```python
from build123d import *


with BuildPart() as part:
    # Sketch → Revolution (revolve)
    with BuildSketch(Plane.XY):
        Polygon((-28.515713, 196), (28.515713, 196), (65.398537, 196), (73.283608, 201), (108, 201), (108, 216), (100, 216), (100, 207), (72.030521, 207), (63.161045, 201.026306), (-29.824583, 201.026306), (-78.099873, 201.026306), (-86.908587, 207), (-100, 207), (-100, 216), (-108, 216), (-108, 201), (-99.298126, 201), (-89.018097, 201), (-80.451416, 196), align=None)
    revolve(axis=Axis((0, 0, 0), (1, 0, 0)))

    # Sketch001 → Revolution001 (revolve)
    with BuildSketch(Plane.XZ):
        with BuildLine():
            Line((0, 0), (100.38707, 0))
            Line((100.38707, 0), (100.38707, 50.972863))
            ThreePointArc((100.38707, 50.972863), (98.816025, 73.680404), (89.94216, 94.641203))
            ThreePointArc((108.836403, 213.905151), (73.659034, 158.34946), (89.94216, 94.641203))
            Line((108.836403, 213.905151), (62.693928, 197.37645))
            Line((62.693928, 197.37645), (29.636631, 197.37645))
            ThreePointArc((29.636631, 197.37645), (34.494433, 122.49617), (51.28, 49.36))
            Line((51.28, 49.36), (0, 49.36))
            Line((0, 49.36), (0, 0))
        make_face()
    revolve(axis=Axis((0, 0, 0), (1, 0, 0)))


solid = part.part
```
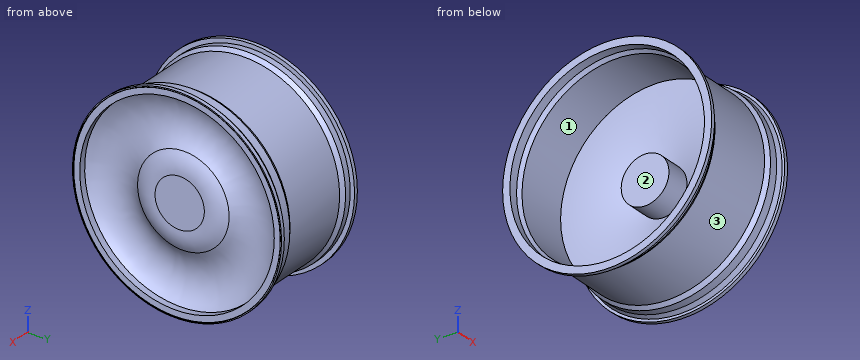
Model file for the job. Use its own axes, mm. Face numbers are marked on the shaded views. Round coordinates to 2 decimals unless told otherwise and drop trailing zeros. Loops run counter-clockwise (first coordinate to the right, second up) from the corner with the lowest first, then second, coordinate; pieces in that order, holes last. Notation, with made-up numbers: M 7.25,24.25 L 56.25,24.25 A22 ccw 56.25,58.25 Z; hole C 15,29 d2. An arc over 180 degrees is marked long. Put each result on its own line as item: value. Start each with the question number.
Item 1: Cut at A-A (x = -8.5). List the corners of the cut face in (y, z), then the cut area to 3 significant figures.
Item 2: Drill centre lines: line 1 along Z through (x, y) = (-95, 0); line 2 along Z through (x, y) = (103.75, 0); line 3 along Y through (x, z) = (-18.5, -141). Where is each one in solid material? Low to high.
Item 3: Drop flat-ended pins along their axis: P1, Ø3, axis at x = 4, z = -41, coming from the +Y side; P2, Ø3, axis at x = -9.5, y = 114.5, coming from the +Z side; P3, Ø2, axis at x = -71, y = -159.5, coming from the -Z side. Give the stop position or say it passes through.
Item 4: Mould opens along Z. For the marked faces 1, 2 and 3 say: released by +Z, released by -Z, zero draft, split by the parting line, or undercut.
Answer block:
1. outline: C 0,0 d402.05; hole C 0,0 d392
1. area: 6,270 mm2
2. line 1: -207 to -201, 201 to 207
2. line 2: -216 to -201, 201 to 216
2. line 3: -143.28 to -136.14, 136.14 to 143.28
3. P1: y = 197.11
3. P2: z = 166.26
3. P3: z = -123.65
4. face 1: undercut
4. face 2: undercut
4. face 3: split by the parting line
